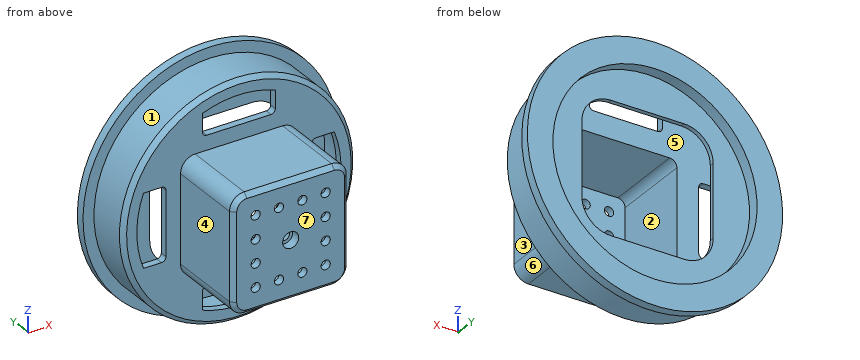
```python
from build123d import *

# Parameters (mm, degrees)
SKETCH1_R                                           = 80
BOSS_EXTRUDE1_DEPTH                                 = 25
SKETCH2_R                                           = 80
SKETCH2_R_2                                         = 70
BOSS_EXTRUDE2_DEPTH                                 = 5
SKETCH3_R                                           = 87.5
SKETCH3_R_2                                         = 70
BOSS_EXTRUDE3_DEPTH                                 = 6
SKETCH5_W                                           = 80
SKETCH5_H                                           = 80
BOSS_EXTRUDE4_DEPTH                                 = 55
SHELL1_START                                        = -50
SHELL1_OUTLINE_W                                    = 70
SHELL1_OUTLINE_H                                    = 70
SHELL1_DEPTH                                        = 75
SHELL1_START_2                                      = 5
SHELL1_2_OUTLINE_R                                  = 75
SHELL1_2_OUTLINE_W                                  = 70
SHELL1_2_OUTLINE_H                                  = 70
SHELL1_2_DEPTH                                      = 20
F_6_3_6_3_DIAMETER_HOLE1_D                          = 6.3
F_6_3_6_3_DIAMETER_HOLE1_DEPTH                      = 10
F_6_3_6_3_DIAMETER_HOLE1_TIP                        = 1.89271095
SKETCH9_R                                           = 5.623813335
BOSS_EXTRUDE5_DEPTH                                 = 5
SKETCH11_R                                          = 70
BOSS_EXTRUDE6_DEPTH                                 = 3
CUT_EXTRUDE2_DEPTH                                  = 6
FILLET2_R                                           = 3
SKETCH18_R                                          = 15.880068884
BOSS_EXTRUDE9_DEPTH                                 = 5
SKETCH19_R                                          = 10
BOSS_EXTRUDE10_DEPTH                                = 10
CBORE_FOR_M6_HEX_SOCKET_HEAD_CAP_SCREW1_D           = 6.6
CBORE_FOR_M6_HEX_SOCKET_HEAD_CAP_SCREW1_CBORE_D     = 11
CBORE_FOR_M6_HEX_SOCKET_HEAD_CAP_SCREW1_CBORE_DEPTH = 6.4
FILLET7_R                                           = 10
FILLET8_R                                           = 5
CHAMFER1_SIZE                                       = 3


# Read off the part's stored shape, not the designer's step: Shell1
with BuildPart() as part:
    # Sketch1 → Boss-Extrude1 (new body)
    with BuildSketch(Plane(origin=(0, 0, 0), x_dir=(1, 0, 0), z_dir=(0, 1, 0))):
        with Locations(Location((0, 0, 0), (0, 0, 270))):
            Circle(SKETCH1_R)
    extrude(amount=BOSS_EXTRUDE1_DEPTH)

    # Sketch2 → Boss-Extrude2 (add)
    with BuildSketch(Plane(origin=(0, 25, 0), x_dir=(1, 0, 0), z_dir=(0, 1, 0))):
        with Locations(Location((0, 0, 0), (0, 0, 270))):
            Circle(SKETCH2_R)
        with Locations(Location((0, 0, 0), (0, 0, 270))):
            Circle(SKETCH2_R_2, mode=Mode.SUBTRACT)
    extrude(amount=BOSS_EXTRUDE2_DEPTH)

    # Sketch3 → Boss-Extrude3 (add)
    with BuildSketch(Plane(origin=(0, 30, 0), x_dir=(1, 0, 0), z_dir=(0, 1, 0))):
        with Locations(Location((0, 0, 0), (0, 0, 270))):
            Circle(SKETCH3_R)
        with Locations(Location((0, 0, 0), (0, 0, 270))):
            Circle(SKETCH3_R_2, mode=Mode.SUBTRACT)
    extrude(amount=BOSS_EXTRUDE3_DEPTH)

    # Sketch5 → Boss-Extrude4 (add)
    with BuildSketch(Plane.XZ):
        Rectangle(SKETCH5_W, SKETCH5_H)
    extrude(amount=BOSS_EXTRUDE4_DEPTH)

    # Shell1 outline → Shell1 (cut)
    with BuildSketch(Plane(origin=(0, 0, 0), x_dir=(1, 0, 0), z_dir=(0, 1, 0)).offset(SHELL1_START)):
        Rectangle(SHELL1_OUTLINE_W, SHELL1_OUTLINE_H)
    extrude(amount=SHELL1_DEPTH, mode=Mode.SUBTRACT)

    # Shell1 2 outline → Shell1 2 (cut)
    with BuildSketch(Plane(origin=(0, 0, 0), x_dir=(1, 0, 0), z_dir=(0, 1, 0)).offset(SHELL1_START_2)):
        Circle(SHELL1_2_OUTLINE_R)
        Rectangle(SHELL1_2_OUTLINE_W, SHELL1_2_OUTLINE_H, mode=Mode.SUBTRACT)
    extrude(amount=SHELL1_2_DEPTH, mode=Mode.SUBTRACT)

    # Ø6.3 (6.3) Diameter Hole1
    with Locations(Plane(origin=(0, -50, 0), x_dir=(1, 0, 0), z_dir=(0, 1, 0))):
        with Locations((0, 0), (24, -24), (-24, 24), (-24, -24), (24, 24), (8, -8), (-8, 8), (-8, -8), (8, 8), (8, 24), (24, 8), (-8, 24), (-24, 8), (-24, -8), (-8, -24), (8, -24), (24, -8)):
            Hole(F_6_3_6_3_DIAMETER_HOLE1_D / 2, depth=F_6_3_6_3_DIAMETER_HOLE1_DEPTH)
            with Locations((0, 0, -(F_6_3_6_3_DIAMETER_HOLE1_DEPTH + F_6_3_6_3_DIAMETER_HOLE1_TIP / 2))):  # 118° drill point
                Cone(0, F_6_3_6_3_DIAMETER_HOLE1_D / 2, F_6_3_6_3_DIAMETER_HOLE1_TIP, mode=Mode.SUBTRACT)

    # Sketch9 → Boss-Extrude5 (add)
    with BuildSketch(Plane(origin=(0, -50, 0), x_dir=(1, 0, 0), z_dir=(0, 1, 0))):
        Circle(SKETCH9_R)
    extrude(amount=-BOSS_EXTRUDE5_DEPTH)

    # Sketch11 → Boss-Extrude6 (add)
    with BuildSketch(Plane(origin=(0, 25, 0), x_dir=(1, 0, 0), z_dir=(0, 1, 0))):
        with Locations(Location((0, 0, 0), (0, 0, 270))):
            Circle(SKETCH11_R)
        with BuildLine():
            Line((-45, 25), (-45, -25))
            ThreePointArc((-45, -25), (-39.142135624, -39.142135624), (-25, -45))
            Line((-25, -45), (25, -45))
            ThreePointArc((25, -45), (39.142135624, -39.142135624), (45, -25))
            Line((45, -25), (45, 25))
            ThreePointArc((45, 25), (39.142135624, 39.142135624), (25, 45))
            Line((25, 45), (-25, 45))
            ThreePointArc((-25, 45), (-39.142135624, 39.142135624), (-45, 25))
        make_face(mode=Mode.SUBTRACT)
    extrude(amount=BOSS_EXTRUDE6_DEPTH)

    # Sketch12 → Cut-Extrude2 (cut)
    with BuildSketch(Plane.XZ):
        with BuildLine():
            Line((-50, 25), (-65.383484153, 25))
            ThreePointArc((-65.383484153, 25), (-70, 0), (-65.383484153, -25))
            Line((-65.383484153, -25), (-50, -25))
            Line((-50, -25), (-50, 25))
        make_face()
        with BuildLine():
            Line((-25, 50), (-25, 65.383484153))
            ThreePointArc((-25, 65.383484153), (0, 70), (25, 65.383484153))
            Line((25, 65.383484153), (25, 50))
            Line((25, 50), (-25, 50))
        make_face()
        with BuildLine():
            Line((50, 25), (65.383484153, 25))
            ThreePointArc((65.383484153, 25), (70, 0), (65.383484153, -25))
            Line((65.383484153, -25), (50, -25))
            Line((50, -25), (50, 25))
        make_face()
        with BuildLine():
            Line((25, -50), (-25, -50))
            Line((-25, -50), (-25, -65.383484153))
            ThreePointArc((-25, -65.383484153), (0, -70), (25, -65.383484153))
            Line((25, -65.383484153), (25, -50))
        make_face()
    extrude(amount=-CUT_EXTRUDE2_DEPTH, mode=Mode.SUBTRACT)

    # Fillet2
    fillet2_edges = [part.edges().sort_by_distance(p)[0] for p in [
        (-50, 2.5, 25),
        (-50, 2.5, -25),
        (25, 2.5, 50),
        (-25, 2.5, 50),
        (50, 2.5, -25),
        (50, 2.5, 25),
        (-25, 2.5, -50),
        (25, 2.5, -50),
    ]]
    fillet(fillet2_edges, radius=FILLET2_R)

    # Sketch18 → Boss-Extrude9 (add)
    with BuildSketch(Plane.XZ.offset(55)):
        Circle(SKETCH18_R)
    extrude(amount=-BOSS_EXTRUDE9_DEPTH)

    # Sketch19 → Boss-Extrude10 (add)
    with BuildSketch(Plane.XZ.offset(55)):
        with Locations(Location((0, 0, 0), (0, 0, 270))):
            Circle(SKETCH19_R)
    extrude(amount=-BOSS_EXTRUDE10_DEPTH)

    # CBORE for M6 Hex Socket Head Cap Screw1 (through all)
    with Locations(Plane(origin=(0, -55, 0), x_dir=(-1, 0, 0), z_dir=(0, -1, 0))):
        with Locations((0, 0)):
            CounterBoreHole(CBORE_FOR_M6_HEX_SOCKET_HEAD_CAP_SCREW1_D / 2, CBORE_FOR_M6_HEX_SOCKET_HEAD_CAP_SCREW1_CBORE_D / 2, CBORE_FOR_M6_HEX_SOCKET_HEAD_CAP_SCREW1_CBORE_DEPTH)

    # Fillet7
    fillet7_edges = [part.edges().sort_by_distance(p)[0] for p in [
        (40, -27.5, -40),
        (40, -27.5, 40),
        (-40, -27.5, 40),
        (-40, -27.5, -40),
    ]]
    fillet(fillet7_edges, radius=FILLET7_R)

    # Fillet8
    fillet8_edges = [part.edges().sort_by_distance(p)[0] for p in [
        (35, -22.5, -35),
        (35, -22.5, 35),
        (-35, -22.5, 35),
        (-35, -22.5, -35),
    ]]
    fillet(fillet8_edges, radius=FILLET8_R)

    # Chamfer1
    chamfer1_edges = [part.edges().sort_by_distance(p)[0] for p in [
        (0, 0, -80),
        (0, -55, -40),
        (-40, -55, 0),
        (40, -55, 0),
        (0, -55, 40),
        (-37.071067812, -55, 37.071067812),
        (37.071067812, -55, 37.071067812),
        (37.071067812, -55, -37.071067812),
        (-37.071067812, -55, -37.071067812),
    ]]
    chamfer(chamfer1_edges, length=CHAMFER1_SIZE)


solid = part.part
```
The model under review builds one solid part; all positions refer to its coordinate system, in mm. Face numbers are marked on the shaded views. A direction names the side the tool comes from. Give positions to 0.01 mm unless a question says otherwise; leave off trailing zeros. Write each loop counter-clockwise with the first axis right and the second up, starting at its lowest first coordinate (ties: lowest second). Pieces come first, ordered by that corner, then holes.
(1) Consider section A-A, the plane y = -19. Give the boundary of the cut face in (x, z).
(2) Tool access review of the marked faces 1, 2, 3 and 4: name each direction out of +Z, -Z, +X, -X, +Y, -Y from which nothing blocks a thin tool from reaching the whole face with its end or side.
(3) Consider section B-B, the plane x = 0. Give the number of separate pieces and of enclosed holes in the cut face, and give its area (3 significant figures).
(4) The part is to be moulded in two halves that separate along Y. For the marked faces 5, 6 and 7, say which applies: released by +Y, released by -Y, zero draft, split by the parting line, or undercut.
(5) To check wall thickness, follow L1, parallel to Z at x = -24, y = -51.85; L2, parallel to X at y = -40.5, z = 23.5; L3, parallel to Y at x = 29.5, z = 54. State the ranges of each line that lie inside material, in increasing order.
(6) For P1, Ø2.5, axis at y = 26, z = -1.5, coming from the -X side; P2, Ø1.5, axis at y = -31.5, z = -31, coming from the -X side; P3, Ø10, axis at x = -18.5, y = 1, coming from the +Z side, all flat-tipped, find the tip position at first contact; note any pin that passes through.
Returned:
1. outline: (-40, -30) arc R10 ccw to (-30, -40) - (30, -40) arc R10 ccw to (40, -30) - (40, 30) arc R10 ccw to (30, 40) - (-30, 40) arc R10 ccw to (-40, 30) - close; hole (-35, -30) arc R5 ccw to (-30, -35) - (30, -35) arc R5 ccw to (35, -30) - (35, 30) arc R5 ccw to (30, 35) - (-30, 35) arc R5 ccw to (-35, 30) - close
2. face 1: -Y
2. face 2: +Y
2. face 3: +Z, -Z, +X, -Y
2. face 4: +Z, -Z, -X, -Y
3. separate pieces: 4
3. enclosed holes: 0
3. area: 1,800 mm2
4. face 5: undercut
4. face 6: zero draft
4. face 7: released by -Y
5. L1: z = -40 to -27.15, -20.85 to -11.15, -4.85 to 4.85, 11.15 to 20.85, 27.15 to 40
5. L2: x = -40 to -35, 35 to 40
5. L3: y = 0 to 5, 25 to 28
6. P1: stops at x = -80
6. P2: stops at x = -40
6. P3: stops at z = 78.78
